Work out the finished part from the listing and answer in its coordinate system (mm). Round coordinates to 2 decimals unless told otherwise and drop trailing zeros. Loops run counter-clockwise (first coordinate to the right, second up) from the corner with the lowest first, then second, coordinate; pieces in that order, holes last. Notation, with made-up numbers: (34, 23.5) -> (40, 23.5) arc R24 cw to (40, 46.5) -> close; hole circle Ø2 at (50, -13). An arc over 180 degrees is marked (long way). Use one line per item in the form item = value.
Autodesk Inventor part; units mm, degrees
ref_plane "YZ Plane" through (0, 0, 0) normal (1, 0, 0) x (0, 1, 0)
ref_plane "XZ Plane" through (0, 0, 0) normal (0, 1, 0) x (-1, 0, 0)
ref_plane "XY Plane" through (0, 0, 0) normal (0, 0, 1) x (1, 0, 0)
sketch "Skizze1" plane through (0, 0, 0) normal (0, 0, 1) x (1, 0, 0)
  circle A0 centre (0, 0) radius 3
  circle A1 centre (0, 0) radius 6
  dimension "d0" = 6
  dimension "d1" = 12
extrude "Extrusion1" add sketch "Skizze1" along normal mid plane 1.6
fillet "Rundung1" radius 0.25 4 edges at (-6, 0, 0.8) (-6, 0, -0.8) (-3, 0, 0.8) (-3, 0, -0.8)
properties part number "900-80-WASHERS-ISO8738-8" material "Edelstahl"
(1) Find section C-C, the plane z = -0.25. Write down the section's boundary in (x, y).
Completed:
outline = circle Ø12 at (0, 0); hole circle Ø6 at (0, 0)
(2) Given P1, Ø5, axis at x = 1.5, y = -1.5, coming from the -Z side, flat-ended and moving along its own axis, determine where the tip first touches the part or whether it passes through.
Completed:
P1 = -0.8
(3) For a pull along Y with two mould halves and no side action, classify faces 1 (the cylindrical face through (-3, 0, 0)), 2 (the flat face through (2.5, -2.5, 0.8)), 3 (the cylindrical face through (-6, 0, 0)) as +Y half, -Y half, draft (parallel to the pull), parting line (faces both ways), or undercut.
Completed:
face_1 = undercut
face_2 = draft
face_3 = parting line
(4) Consider L1, parallel to Y at x = 0, z = 0; L2, parallel to X at y = 2.5, z = 0.4; L3, parallel to X at y = 1.5, z = -0.7. Determine where each line is inside the solid, lowest interval first.
Completed:
L1 = -6 to -3, 3 to 6
L2 = -5.45 to -1.66, 1.66 to 5.45
L3 = -5.76 to -2.66, 2.66 to 5.76
(5) Find section A-A, the plane x = 0. Write down the section's boundary in (y, z), then the cut area to 3 significant figures.
Completed:
outline = (-6, -0.55) arc R0.25 ccw to (-5.75, -0.8) -> (-3.25, -0.8) arc R0.25 ccw to (-3, -0.55) -> (-3, 0.55) arc R0.25 ccw to (-3.25, 0.8) -> (-5.75, 0.8) arc R0.25 ccw to (-6, 0.55) -> close; (3, -0.55) arc R0.25 ccw to (3.25, -0.8) -> (5.75, -0.8) arc R0.25 ccw to (6, -0.55) -> (6, 0.55) arc R0.25 ccw to (5.75, 0.8) -> (3.25, 0.8) arc R0.25 ccw to (3, 0.55) -> close
area = 9.49 mm2
